For this review, take the finished solid that the model builds, in its own axes (mm). Face numbers are marked on the shaded views. A direction names the side the tool comes from. Round coordinates to 2 decimals unless told otherwise and drop trailing zeros. Write each loop counter-clockwise with the first axis right and the second up, starting at its lowest first coordinate (ties: lowest second). Pieces come first, ordered by that corner, then holes. Notation, with made-up numbers: (89.25, 37.25) - (98.25, 37.25) arc R23 ccw to (98.25, 73.25) - close; hole circle Ø8 at (-15.75, 37). An arc over 180 degrees is marked (long way). Answer in a Markdown table with one row per item. Add a question column.
from build123d import *

# Parameters (mm, degrees)
F1_DEPTH = 15
F0_W     = 25
F0_H     = 20
F2_DEPTH = 5


with BuildPart() as f1:
    # F0 (on Top) → F1 (new body)
    with BuildSketch(Plane.XY):
        with BuildLine():
            ThreePointArc((12.5, -11), (23.5, 0), (12.5, 11))
            Line((12.5, 11), (-13.5, 11))
            Line((-13.5, 11), (-13.5, -11))
            Line((-13.5, -11), (12.5, -11))
        make_face()
        with BuildLine():
            Line((-12.5, 10), (12.5, 10))
            ThreePointArc((12.5, 10), (22.5, 0), (12.5, -10))
            Line((12.5, -10), (-12.5, -10))
            Line((-12.5, -10), (-12.5, 10))
        make_face(mode=Mode.SUBTRACT)
    extrude(amount=F1_DEPTH)

    # F0 (on Top) → F2 (join)
    with BuildSketch(Plane.XY):
        Rectangle(F0_W, F0_H)
        with BuildLine():
            ThreePointArc((12.5, -10), (22.5, 0), (12.5, 10))
            Line((12.5, 10), (12.5, -10))
        make_face()
    extrude(amount=F2_DEPTH)


solid = f1.part
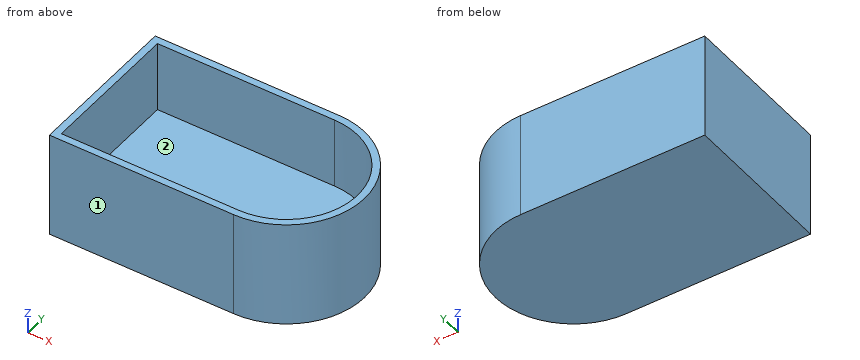
Q1. Add section B-B on y = 0. State the section outline as (x, z) points, then the cut area to 3 significant figures.
Q2. Insertion check: pin 1 Ø1 at (x, y) = (-4.5, -4.5) entering from +Z; pin 2 Ø2 at (y, z) = (-3, 3) entering from +X. Each pin has a flat end and moves straight along its axis. Give the tip position at first contact, or say it passes through.
Q3. Add section C-C on x = -5.5. State the section outline as (y, z) points.
Q4. To check wall thickness, follow probe 1 along Y at (x, z) = (3, 6.5); probe 2 along Z at (x, y) = (8, -7.25); probe 3 along Y at (x, z) = (14.5, 7). State the ranges of each line that lie inside material, in increasing order.
Q5. Tool access review of the marked faces 1 and 2: name each direction out of +Z, -Z, +X, -X, +Y, -Y from which nothing blocks a thin tool from reaching the whole face with its end or side.
Q6. Add section A-A on z = 12. State the section outline as (x, y) points, then the cut area to 3 significant figures.
Answer sheet:
| question | item | result |
|---|---|---|
| 1 | outline | (-13.5, 0) - (23.5, 0) - (23.5, 15) - (22.5, 15) - (22.5, 5) - (-12.5, 5) - (-12.5, 15) - (-13.5, 15) - close |
| 1 | area | 205 mm² |
| 2 | pin 1 | stops at z = 5 |
| 2 | pin 2 | stops at x = 23.32 |
| 3 | outline | (-11, 0) - (11, 0) - (11, 15) - (10, 15) - (10, 5) - (-10, 5) - (-10, 15) - (-11, 15) - close |
| 4 | probe 1 | y = -11 to -10, 10 to 11 |
| 4 | probe 2 | z = 0 to 5 |
| 4 | probe 3 | y = -10.82 to -9.8, 9.8 to 10.82 |
| 5 | face 1 | +Z, -Z, +X, -X, -Y |
| 5 | face 2 | +Z |
| 6 | outline | (-13.5, -11) - (12.5, -11) arc R11 ccw to (12.5, 11) - (-13.5, 11) - close; hole (-12.5, -10) - (12.5, -10) arc R10 ccw to (12.5, 10) - (-12.5, 10) - close |
| 6 | area | 105 mm² |
